```python
from build123d import *

# Parameters (mm, degrees)
BOSS_EXTRUDE1_DEPTH = 6
SKETCH3_W           = 6
SKETCH3_H           = 12
BOSS_EXTRUDE2_DEPTH = 6


with BuildPart() as part:
    # Sketch2 → Boss-Extrude1 (new body)
    with BuildSketch(Plane.XY):
        Polygon((-66, 6), (-78, 6), (-78, 0), (-90, 0), (-90, 6), (-102.5, 6), (-102.5, -65.99938194), (-90, -65.99938194), (-90, -59.99938194), (-78, -59.99938194), (-78, -65.99938194), (-66, -65.99938194), (-66, -59.99938194), (-54, -59.99938194), (-54, -65.99938194), (-42, -65.99938194), (-42, -59.99938194), (-30, -59.99938194), (-30, -65.99938194), (-18, -65.99938194), (-18, -59.99938194), (-6, -59.99938194), (-6, -65.99938194), (6, -65.99938194), (6, -59.99938194), (18, -59.99938194), (18, -65.99938194), (30, -65.99938194), (30, -59.99938194), (42, -59.99938194), (42, -65.99938194), (54, -65.99938194), (54, -59.99938194), (66, -59.99938194), (66, -65.99938194), (78, -65.99938194), (78, -59.99938194), (90, -59.99938194), (90, -65.99938194), (102.5, -65.99938194), (102.5, 6), (90, 6), (90, 0), (78, 0), (78, 6), (66, 6), (66, 0), (54, 0), (54, 6), (42, 6), (42, 0), (30, 0), (30, 6), (18, 6), (18, 0), (6, 0), (6, 6), (-6, 6), (-6, 0), (-18, 0), (-18, 6), (-30, 6), (-30, 0), (-42, 0), (-42, 6), (-54, 6), (-54, 0), (-66, 0), align=None)
    extrude(amount=BOSS_EXTRUDE1_DEPTH)

    # Sketch3 → Boss-Extrude2 (add)
    with BuildSketch(Plane.XY.offset(6)):
        with Locations((-105.5, -6)):
            Rectangle(SKETCH3_W, SKETCH3_H)
        with Locations((105.5, -6)):
            Rectangle(SKETCH3_W, SKETCH3_H)
        with Locations((105.5, -30)):
            Rectangle(SKETCH3_W, SKETCH3_H)
        with Locations((105.5, -54)):
            Rectangle(SKETCH3_W, SKETCH3_H)
        with Locations((-105.5, -30)):
            Rectangle(SKETCH3_W, SKETCH3_H)
        with Locations((-105.5, -54)):
            Rectangle(SKETCH3_W, SKETCH3_H)
    extrude(amount=-BOSS_EXTRUDE2_DEPTH)


solid = part.part
```
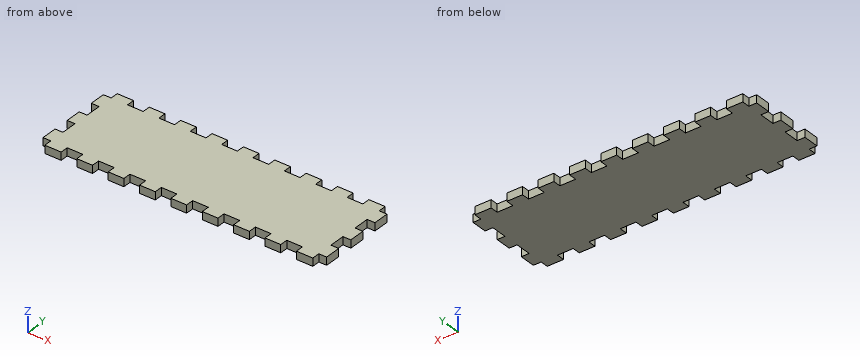
Build history of the part. All positions in model axes, mm. Round coordinates to 2 decimals unless told otherwise and drop trailing zeros. Order: outer loops, then holes, each group sorted by start corner. A loop starts at its lowest first (then second) coordinate and runs counter-clockwise, first axis right, second up. Notation, with made-up numbers: (85.5, 40) - (127.5, 40) arc R26 ccw to (127.5, 57) - close; hole circle Ø2 at (22.25, 47.25). An arc over 180 degrees is marked (long way). Use a Markdown table: item, result.
1) Saw through at A-A on y = -42. Write the cut outline in (x, z), and give its area (3 significant figures).
Recorded:
| item | result |
|---|---|
| outline | (-102.5, 0) - (102.5, 0) - (102.5, 6) - (-102.5, 6) - close |
| area | 1,230 mm² |
2) Saw through at B-B on x = 87. Write the cut outline in (y, z).
Recorded:
| item | result |
|---|---|
| outline | (-60, 0) - (0, 0) - (0, 6) - (-60, 6) - close |
3) Wall check: L1, parallel to X at y = -45, z = 0.65; L2, parallel to Y at x = -65, z = 4.5. Give the ranges that are in metal, low to high.
Recorded:
| item | result |
|---|---|
| L1 | x = -102.5 to 102.5 |
| L2 | y = -60 to 0 |
4) Flat gauge pins, fed straight in: pin 1 Ø1.8 at (y, z) = (-61.5, 4.5) entering from +X; pin 2 Ø3 at (y, z) = (-62, 3) entering from -X; pin 3 Ø1 at (x, z) = (-10.5, 3) entering from -Y. Where does each tip first touch, or does it go through?
Recorded:
| item | result |
|---|---|
| pin 1 | stops at x = 102.5 |
| pin 2 | stops at x = -102.5 |
| pin 3 | stops at y = -60 |
